The drawing under review shows one solid part. Ordinate dimensions are in mm from its lowest x, y, z. A direction names the side the tool comes from. Give positions to 0.01 mm unless a question says otherwise; leave off trailing zeros. Write each loop counter-clockwise with the first axis right and the second up, starting at its lowest first coordinate (ties: lowest second). Pieces come first, ordered by that corner, then holes. Notation, with made-up numbers: (24, -37) -> (80, -37) arc R5 cw to (80, -30) -> close; hole circle Ø1 at (84.25, 18). An arc over 180 degrees is marked (long way). Answer as a JSON object with one key per item and string values.
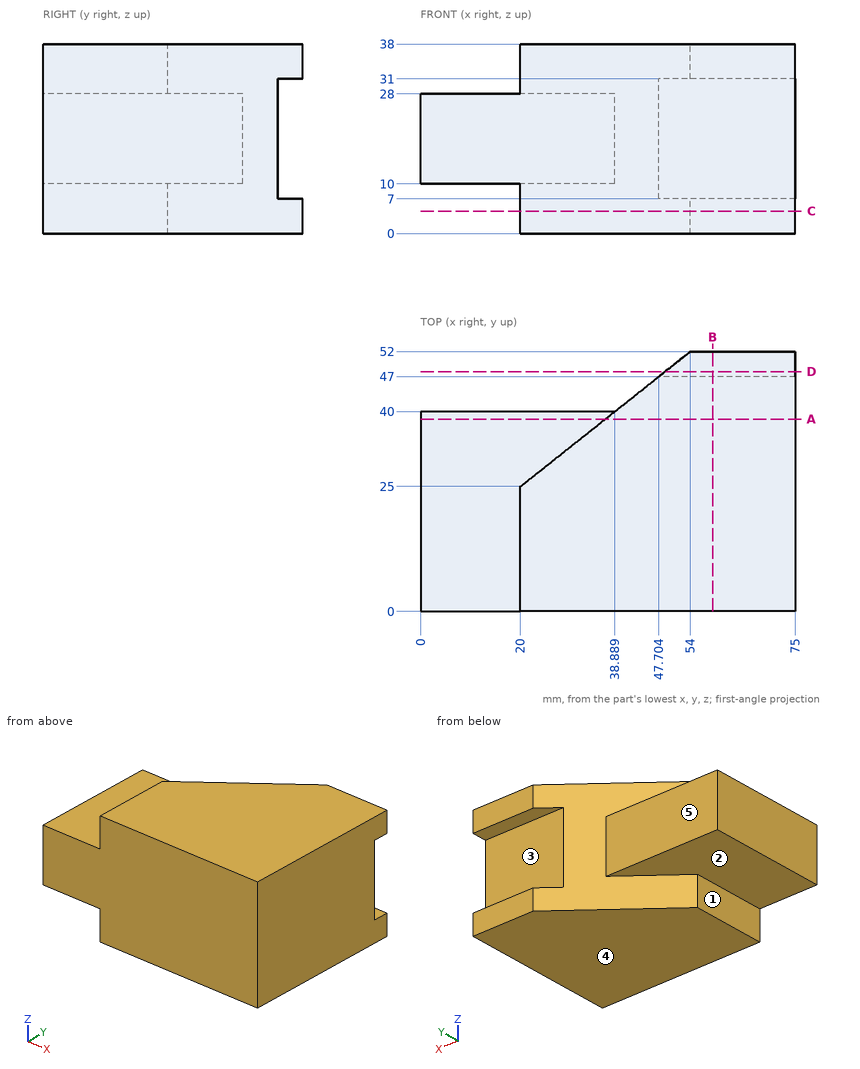
(1) We need section B-B, the plane x = 58.5. State the section outline as (y, z) points.
Here are the results:
{"outline": "(0, 0) -> (52, 0) -> (52, 7) -> (47, 7) -> (47, 31) -> (52, 31) -> (52, 38) -> (0, 38) -> close"}
(2) For line 1 along X through (y, z) = (17, 29); line 2 along Y through (x, z) = (27, 23); line 3 along Y through (x, z) = (59.5, 23), list the stretches that pass through material, from the lowest coordinate up.
Here are the results:
{"line 1": "x = 20 to 75", "line 2": "y = 0 to 40", "line 3": "y = 0 to 47"}
(3) We need section D-D, the plane y = 48. State the section outline as (x, z) points.
Here are the results:
{"outline": "(48.96, 0) -> (75, 0) -> (75, 7) -> (48.96, 7) -> close; (48.96, 31) -> (75, 31) -> (75, 38) -> (48.96, 38) -> close"}
(4) Clearance check with flat-ended pins moving along their axes: pin 1 (1 mm diameter, centred on x = 30.5, z = 32.5, fed in from +Y) (1 decimal); pin 2 (14.5 mm diameter, centred on x = 24, z = 21.5, fed in from +Y); pin 3 (10 mm diameter, centred on x = 61, z = 18.5, fed in from +Y). State where each tip first meets the part, or that it passes through.
Here are the results:
{"pin 1": "stops at y = 33.7", "pin 2": "stops at y = 40", "pin 3": "stops at y = 47"}
(5) We need section C-C, the plane z = 4.5. State the section outline as (x, y) points, then the cut area to 3 significant figures.
Here are the results:
{"outline": "(20, 0) -> (75, 0) -> (75, 52) -> (54, 52) -> (20, 25) -> close", "area": "2,400 mm²"}
(6) For the marked faces 4 and 5, list the 3-axis set-ups (+Z, -Z, +X, -X, +Y, -Y) from which the entire face can be reached by the end or side of a thin tool; tool diameter is ignored.
Here are the results:
{"face 4": "-Z, +X, -X, +Y, -Y", "face 5": "+Z, -Z, -X, +Y"}
(7) The part is to be moulded in two halves that separate along Z. For the marked faces 1, 2 and 3, say which applies: +Z half, -Z half, draft (parallel to the pull), parting line (faces both ways), or undercut.
Here are the results:
{"face 1": "draft", "face 2": "-Z half", "face 3": "undercut"}
(8) We need section A-A, the plane y = 38.5. State the section outline as (x, z) points.
Here are the results:
{"outline": "(0, 10) -> (37, 10) -> (37, 0) -> (75, 0) -> (75, 38) -> (37, 38) -> (37, 28) -> (0, 28) -> close"}
